For this review, take the finished solid that the model builds, in its own axes (mm). A direction names the side the tool comes from. Coordinates: 2 decimals unless noted, no trailing zeros. Order: outer loops, then holes, each group sorted by start corner. A loop starts at its lowest first (then second) coordinate and runs counter-clockwise, first axis right, second up. Notation, with made-up numbers: (-5.5, 17.25) -> (37.5, 17.25) arc R22 cw to (37.5, 34.25) -> close; hole circle Ø3 at (48.5, -40). An arc over 180 degrees is marked (long way). Answer as a JSON object with one key per item and string values. Group by question number.
1) Add section A-A, the plane y = -23. Write out the cut boundary in (x, z).
2) Draft analysis for pull direction Z (two halves, no side actions). For faces 4 (the flat face through (-5, -35.56, 1)), 5 (the flat face through (-5, -18, 57.15)), 6 (the flat face through (-363.47, -18.03, 34.93)), state which applies: +Z half, -Z half, draft (parallel to the pull), parting line (faces both ways), or undercut.
3) For pin 1 (10 mm diameter, centred on y = -22.5, z = 26.5, fed in from -X); pin 2 (4 mm diameter, centred on y = -21.5, z = -10.5, fed in from +X), all flat-tipped, find the tip position at first contact; note any pin that passes through.
4) Wall thickness on L1, parallel to X at y = -34, z = 37.5: over which ranges is the line inside the solid? List them lowest first.
5) Add section B-B, the plane z = 2. Write out the cut boundary in (x, y).
6) Machinability: for faces 1 (the flat face through (363.47, -18.03, -34.93)), 2 (the flat face through (-5, 0, 1)), 3 (the flat face through (-363.47, -17.53, -34.84)), which of the approach directions +Z, -Z, +X, -X, +Y, -Y give a long, thin tool a straight path to every point of the face, cutting with its end or side? Answer none if there is none.
from build123d import *

# Parameters (mm, degrees)
F0_W     = 762
F0_H     = 114.3
F1_DEPTH = 35.56
F3_DEPTH = 35.56
F5_DEPTH = 35.56


with BuildPart() as f1:
    # F0 (on Front) → F1 (new body)
    with BuildSketch(Plane.XZ):
        Rectangle(F0_W, F0_H)
    extrude(amount=F1_DEPTH)

    # F2 (on face) → F3 (cut)
    with BuildSketch(Plane(origin=(-381, 0, 0), x_dir=(0, -1, 0), z_dir=(-1, 0, 0))):
        Polygon((35.56, 38.020187), (0, 31.75), (0, -31.75), (35.56, -38.020187), align=None)
    extrude(amount=-F3_DEPTH, mode=Mode.SUBTRACT)

    # F4 (on face) → F5 (cut)
    with BuildSketch(Plane.YZ.offset(381)):
        Polygon((0, 31.75), (-35.56, 38.020187), (-35.56, -38.020187), (0, -31.75), align=None)
    extrude(amount=-F5_DEPTH, mode=Mode.SUBTRACT)


solid = f1.part
Output values:
{
 "1": {"outline": "(-381, -57.15) -> (381, -57.15) -> (381, -35.81) -> (345.44, -35.81) -> (345.44, 35.81) -> (381, 35.81) -> (381, 57.15) -> (-381, 57.15) -> (-381, 35.81) -> (-345.44, 35.81) -> (-345.44, -35.81) -> (-381, -35.81) -> close"},
 "2": {"face 4": "draft", "face 5": "+Z half", "face 6": "undercut"},
 "3": {"pin 1": "stops at x = -345.44", "pin 2": "stops at x = 345.44"},
 "4": {"L1": "x = -345.44 to 345.44"},
 "5": {"outline": "(-345.44, -35.56) -> (345.44, -35.56) -> (345.44, 0) -> (-345.44, 0) -> close"},
 "6": {"face 1": "+X, -Y", "face 2": "+Z, -Z, +X, -X, +Y", "face 3": "-X, -Y"}
}
